Verification items for the finished model (mm, model axes). Face numbers are marked on the shaded views. A direction names the side the tool comes from. Round coordinates to 2 decimals unless told otherwise and drop trailing zeros. Order: outer loops, then holes, each group sorted by start corner. A loop starts at its lowest first (then second) coordinate and runs counter-clockwise, first axis right, second up. Notation, with made-up numbers: M -32,40.25 L -3,40.25 A23 ccw -3,53.25 Z; hole C 38,-38.75 d11. An arc over 180 degrees is marked long. Answer as a JSON object with one key per item and string values. Group by question number.
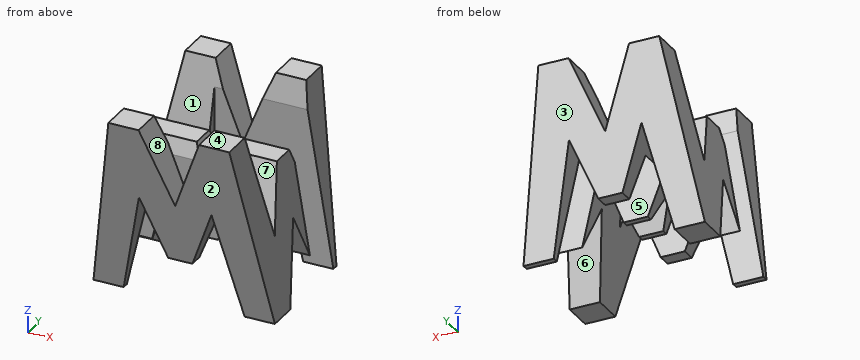
```python
from build123d import *

# Parameters (mm, degrees)
F0_W      = 38.1
F0_H      = 38.1
F1_DEPTH  = 38.1
F6_DEPTH  = 38.1
F8_DEPTH  = 38.1
F9_W      = 24.996
F9_H      = 7.62
F9_W_2    = 25.452001
F10_DEPTH = 38.1


with BuildPart() as f1:
    # F0 (on Front) → F1 (new body)
    with BuildSketch(Plane.XZ):
        with Locations((19.05, 19.05)):
            Rectangle(F0_W, F0_H)
    extrude(amount=F1_DEPTH)

    # F5 (on offset) → F6 (cut)
    with BuildSketch(Plane.YZ.offset(38.1)):
        Polygon((-6.35, 38.1), (-31.75, 38.1), (-26.67, 15.671999), (-21.59, 28.575), (-16.51, 28.575), (-11.43, 16.175999), align=None)
        Polygon((-19.05, 15.875), (-25.4, 0), (-12.7, 0), align=None)
        Polygon((-31.75, 0), (-38.1, 38.1), (-38.1, 0), align=None)
        Polygon((0, 0), (0, 38.1), (-6.35, 0), align=None)
    extrude(amount=-F6_DEPTH, mode=Mode.SUBTRACT)

    # F7 (on offset) → F8 (cut)
    with BuildSketch(Plane.XZ.offset(38.1)):
        Polygon((25.4, 38.1), (12.7, 38.1), (19.05, 22.225), align=None)
        Polygon((0, 38.1), (0, 0), (6.35, 38.1), align=None)
        Polygon((11.43, 22.225), (6.35, 0), (31.75, 0), (26.67, 22.225), (21.59, 9.525), (16.51, 9.525), align=None)
        Polygon((31.75, 38.1), (38.1, 0), (38.1, 38.1), align=None)
    extrude(amount=-F8_DEPTH, mode=Mode.SUBTRACT)

    # F9 (on offset) → F10 (cut)
    with BuildSketch(Plane.XY.offset(38.1)):
        with Locations((25.602, -11.43)):
            Rectangle(F9_W, F9_H)
        with Locations((12.726, -26.67)):
            Rectangle(F9_W_2, F9_H)
    extrude(amount=-F10_DEPTH, mode=Mode.SUBTRACT)


solid = f1.part
```
Q1. Gauge pin test, flat ends, axial feed: pin 1 Ø4 at (x, y) = (30.5, -20.5) entering from +Z (3 decimals); pin 2 Ø3.5 at (y, z) = (-28.5, 27.5) entering from -X; pin 3 Ø0.6 at (x, y) = (20, -22) entering from -Z (3 decimals). Record the tip position at first contact, or that the pin passes through.
Q2. Cross-section at A-A, the plane x = 12. Give the number of separate pieces and of enclosed holes in the cut face, then the cut area to 3 significant figures.
Q3. Release check for a two-part mould opening along Y. For the marked faces 1, 2, 3 and 4 record: released by +Y, released by -Y, zero draft, split by the parting line, or undercut.
Q4. Thickness scan on line 1 (X direction, y = -4, z = 16.5); line 2 (Y direction, x = 10, z = 27); line 3 (X direction, y = -2, z = 28). Record the ranges inside material, lowest first. Write a range as from..to.
Q5. Cross-section at D-D, the plane z = 27.5. Record the cut outline in (x, y).
Q6. Tool access check on the marked faces 5, 6, 7 and 8. Record the directions out of +Z, -Z, +X, -X, +Y, -Y that give a thin tool (end or side, any length) a straight path to the whole face; none if there is none.
Conclusion:
{
 "1": {"pin 1": "z = 28.575", "pin 2": "x = 25.45", "pin 3": "z = 9.525"},
 "2": {"separate pieces": "3", "enclosed holes": "0", "area": "283 mm2"},
 "3": {"face 1": "undercut", "face 2": "released by -Y", "face 3": "released by +Y", "face 4": "zero draft"},
 "4": {"line 1": "2.75..10.12, 13.72..24.38, 27.98..35.35", "line 2": "-36.25..-30.48, -22.21..-15.86, -8.92..-1.85", "line 3": "4.67..16.74, 21.36..33.43"},
 "5": {"outline": "M 4.58,-36.33 L 16.94,-36.33 L 16.94,-30.48 L 4.58,-30.48 Z; M 4.58,-22.01 L 16.94,-22.01 L 16.94,-16.07 L 4.58,-16.07 Z; M 4.58,-8.81 L 13.1,-8.81 L 13.1,-7.62 L 16.94,-7.62 L 16.94,-1.77 L 4.58,-1.77 Z; M 21.16,-36.33 L 33.52,-36.33 L 33.52,-29.35 L 25.45,-29.35 L 25.45,-30.48 L 21.16,-30.48 Z; M 21.16,-22.01 L 33.52,-22.01 L 33.52,-16.07 L 21.16,-16.07 Z; M 21.16,-7.62 L 33.52,-7.62 L 33.52,-1.77 L 21.16,-1.77 Z"},
 "6": {"face 5": "+Z, -Z, +X", "face 6": "-Z, +X, -X", "face 7": "+Z, +X, -X", "face 8": "+Z, +Y, -Y"}
}
